from build123d import *

# Parameters (mm, degrees)
F2_DEPTH      = 25
F4_DEPTH      = 70
F5_R          = 35.5
F6_DEPTH      = 10
F6_DEPTH_BACK = 120
F7_R          = 38.3333333333
F8_DEPTH      = 10
F8_DEPTH_BACK = 120
F9_R          = 20.5
F10_DEPTH     = 223.001
F11_R         = 20.5
F12_DEPTH     = 210.001
F14_DEPTH     = 10


with BuildPart() as f2:
    # F1 (on Top) → F2 (new body)
    with BuildSketch(Plane.XY):
        with BuildLine():
            ThreePointArc((0, 10), (2.9289321881, 2.9289321881), (10, 0))
            Line((10, 0), (190, 0))
            ThreePointArc((190, 0), (197.0710678119, 2.9289321881), (200, 10))
            Line((200, 10), (200, 203))
            ThreePointArc((200, 203), (197.0710678119, 210.0710678119), (190, 213))
            Line((190, 213), (10, 213))
            ThreePointArc((10, 213), (2.9289321881, 210.0710678119), (0, 203))
            Line((0, 203), (0, 10))
        make_face()
    extrude(amount=F2_DEPTH)

    # F3 (on face) → F4 (join)
    with BuildSketch(Plane.XY.offset(25)):
        with BuildLine():
            Line((30, 80), (30, 0))
            Line((30, 0), (45, 0))
            Line((45, 0), (45, 66.0769515459))
            ThreePointArc((45, 66.0769515459), (104.2462120246, 95.7537879754), (133.9230484541, 155))
            Line((133.9230484541, 155), (200, 155))
            Line((200, 155), (200, 170))
            Line((200, 170), (120, 170))
            ThreePointArc((120, 170), (93.6396103068, 106.3603896932), (30, 80))
        make_face()
    extrude(amount=F4_DEPTH)

    # F5 (on face) → F6 (join, two sides)
    with BuildSketch(Plane.XZ) as f6_sk:
        with Locations((37.5, 95)):
            Circle(F5_R)
    extrude(amount=F6_DEPTH)
    extrude(f6_sk.sketch, amount=-F6_DEPTH_BACK)

    # F7 (on face) → F8 (join, two sides)
    with BuildSketch(Plane.YZ.offset(200)) as f8_sk:
        with Locations((162.5, 95)):
            Circle(F7_R)
    extrude(amount=F8_DEPTH)
    extrude(f8_sk.sketch, amount=-F8_DEPTH_BACK)

    # F9 (on face) → F10 (cut, through all)
    with BuildSketch(Plane.XZ.offset(10)):
        with Locations((37.5, 95)):
            Circle(F9_R)
    extrude(amount=-F10_DEPTH, mode=Mode.SUBTRACT)

    # F11 (on face) → F12 (cut, through all)
    with BuildSketch(Plane.YZ.offset(210)):
        with Locations((162.5, 95)):
            Circle(F11_R)
    extrude(amount=-F12_DEPTH, mode=Mode.SUBTRACT)

    # F13 (on face) → F14 (join)
    with BuildSketch(Plane.XY.offset(25)):
        with BuildLine():
            Line((200, 10), (200, 49.6179956198))
            Line((200, 49.6179956198), (164.4239968061, 49.6179956198))
            ThreePointArc((164.4239968061, 49.6179956198), (157.3529289943, 46.6890634316), (154.4239968061, 39.6179956198))
            Line((154.4239968061, 39.6179956198), (154.4239968061, 0))
            Line((154.4239968061, 0), (190, 0))
            ThreePointArc((190, 0), (197.0710678119, 2.9289321881), (200, 10))
        make_face()
    extrude(amount=F14_DEPTH)


solid = f2.part
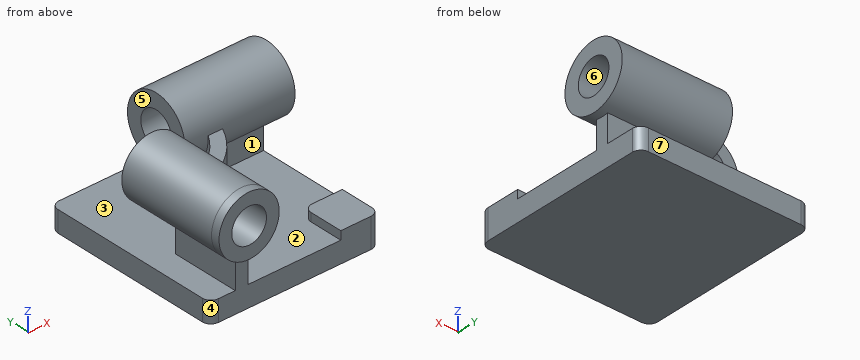
Source: CAD feature listing. Evaluate the final solid. Frame: model axes, mm. Face numbers are marked on the shaded views. A direction names the side the tool comes from. Round coordinates to 2 decimals unless told otherwise and drop trailing zeros. Order: outer loops, then holes, each group sorted by start corner. A loop starts at its lowest first (then second) coordinate and runs counter-clockwise, first axis right, second up. Notation, with made-up numbers: (-13.5, -21.75) - (-6.5, -21.75) arc R28 cw to (-6.5, 11.25) - close; hole circle Ø5 at (12, 37.25). An arc over 180 degrees is marked (long way). Use a Markdown table: item, result. Add a question column.
1. First-contact query: pin 1 (4 mm diameter, centred on x = 127, y = 132.5, fed in from +Z); pin 2 (15 mm diameter, centred on x = 87, y = 94.5, fed in from +Z); pin 3 (2 mm diameter, centred on x = 86, y = 31, fed in from +Z); pin 4 (2 mm diameter, centred on x = 87.5, y = 188, fed in from -Z). Flat tips, straight axial feed; report the tip coordinate or a pass-through.
2. Section query B-B (y = 95). Return the cut outline in (x, z).
3. Section query C-C (x = 37). Return the cut outline in (y, z), then the cut area to 3 significant figures.
4. Set-up query: the marked faces 1, 2, 3 and 4. Return all of +Z, -Z, +X, -X, +Y, -Y with unobstructed straight access to the full face (end or side cutting, diameter ignored); none if empty.
5. Section query D-D (z = 79). Return the cut outline in (x, y), then the cut area to 3 significant figures.
6. Line query: probe 1 along Z at (x, y) = (36, 8.5); probe 2 along Z at (x, y) = (158, 162); probe 3 along X at (y, z) = (48.5, 11.5). Output: solid intervals per line, ascending.
7. Mould query, pull axis Y, two halves, no side actions, for the marked faces 5, 6 and 7. Classes: +Y half, -Y half, draft (parallel to the pull), parting line (faces both ways), or undercut.
8. Section query A-A (x = 85.5). Return the cut outline in (y, z), then the cut area to 3 significant figures.
Derived:
| question | item | result |
|---|---|---|
| 1 | pin 1 | z = 121.18 |
| 1 | pin 2 | z = 95 |
| 1 | pin 3 | z = 25 |
| 1 | pin 4 | z = 0 |
| 2 | outline | (0, 0) - (200, 0) - (200, 25) - (103.48, 25) - (103.48, 95) - (79.75, 95) - (79.75, 25) - (0, 25) - close; circle Ø71 at (37.5, 95); hole circle Ø41 at (37.5, 95) |
| 3 | outline | (-10, 59.5) - (0, 59.5) - (0, 0) - (213, 0) - (213, 25) - (80.27, 25) - (80.27, 59.5) - (120, 59.5) - (120, 74.51) - (-10, 74.51) - close; (-10, 115.49) - (120, 115.49) - (120, 130.5) - (-10, 130.5) - close |
| 3 | area | 12,000 mm2 |
| 4 | face 1 | +X |
| 4 | face 2 | none |
| 4 | face 3 | -X, +Y |
| 4 | face 4 | -Z, -X, -Y |
| 5 | outline | (5.81, -10) - (24.68, -10) - (24.68, 120) - (5.81, 120) - close; (50.32, -10) - (69.19, -10) - (69.19, 72.59) arc R105 ccw to (126.09, 127.67) - (210, 127.67) - (210, 149.68) - (80, 149.68) - (80, 127.67) - (109.42, 127.67) arc R90 cw to (69.19, 88.98) - (69.19, 120) - (50.32, 120) - close; (80, 175.32) - (210, 175.32) - (210, 197.33) - (80, 197.33) - close |
| 5 | area | 11,700 mm2 |
| 6 | probe 1 | 0 to 74.55, 115.45 to 130.47 |
| 6 | probe 2 | 0 to 74.51, 115.49 to 133.33 |
| 6 | probe 3 | 0 to 200 |
| 7 | face 5 | draft |
| 7 | face 6 | undercut |
| 7 | face 7 | +Y half |
| 8 | outline | (0, 0) - (213, 0) - (213, 25) - (99.15, 25) - (99.15, 95) - (80.87, 95) - (80.87, 25) - (0, 25) - close; circle Ø76.67 at (162.5, 95); hole circle Ø41 at (162.5, 95) |
| 8 | area | 9,900 mm2 |
